Build history of the part. All positions in model axes, mm. Give positions to 0.01 mm unless a question says otherwise; leave off trailing zeros. Order: outer loops, then holes, each group sorted by start corner. A loop starts at its lowest first (then second) coordinate and runs counter-clockwise, first axis right, second up. Notation, with made-up numbers: (73, 11.5) - (132, 11.5) arc R8 ccw to (132, 26.5) - close; hole circle Ø2 at (-36.75, -16.5). An arc over 180 degrees is marked (long way). Answer in a Markdown table with one row per item.
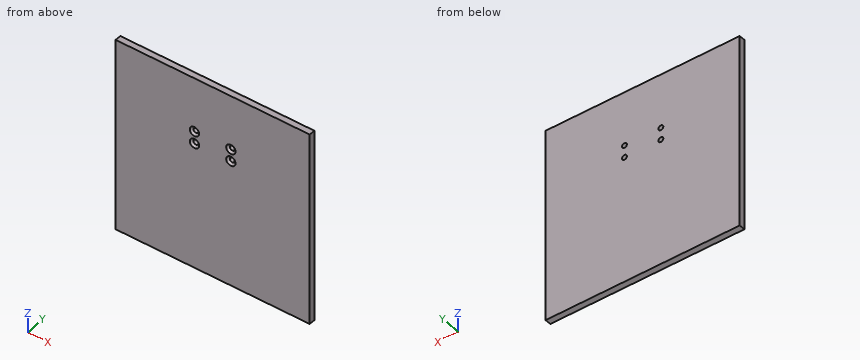
```python
from build123d import *

# Parameters (mm, degrees)
SKETCH2_W                                          = 203.2
SKETCH2_H                                          = 203.2
BOSS_EXTRUDE2_DEPTH                                = 6.35
CSK_FOR_10_FLAT_HEAD_MACHINE_SCREW_100_D           = 5.1054
CSK_FOR_10_FLAT_HEAD_MACHINE_SCREW_100_CSINK_D     = 9.779
CSK_FOR_10_FLAT_HEAD_MACHINE_SCREW_100_CSINK_ANGLE = 100


with BuildPart() as part:
    # Sketch2 → Boss-Extrude2 (new body)
    with BuildSketch(Plane(origin=(0, 0, 0), x_dir=(1, 0, 0), z_dir=(0, 1, 0))):
        with Locations((101.6, 101.6)):
            Rectangle(SKETCH2_W, SKETCH2_H)
    extrude(amount=BOSS_EXTRUDE2_DEPTH)

    # CSK for #10 Flat Head Machine Screw (100)1 (through all)
    with Locations(Plane(origin=(0, 0, 0), x_dir=(-1, 0, 0), z_dir=(0, -1, 0))):
        with Locations((-82.55, 57.15), (-82.55, 69.85), (-120.65, 57.15), (-120.65, 69.85)):
            CounterSinkHole(CSK_FOR_10_FLAT_HEAD_MACHINE_SCREW_100_D / 2, CSK_FOR_10_FLAT_HEAD_MACHINE_SCREW_100_CSINK_D / 2, counter_sink_angle=CSK_FOR_10_FLAT_HEAD_MACHINE_SCREW_100_CSINK_ANGLE)


solid = part.part
```
1. Probe line 1 (Z direction, x = 120.65, y = 4.35); line 2 (X direction, y = 3.4, z = -57.15); line 3 (Z direction, x = 81, y = 3). List the from-to ranges inside material, lowest first.
Check result:
| item | result |
|---|---|
| line 1 | z = -203.2 to -72.4, -67.3 to -59.7, -54.6 to 0 |
| line 2 | x = 0 to 80, 85.1 to 118.1, 123.2 to 203.2 |
| line 3 | z = -203.2 to -71.88, -67.82 to -59.18, -55.12 to 0 |
2. Drop flat-ended pins along their axis: P1, Ø6.5, axis at x = 82.55, z = -69.85, coming from the -Y side; P2, Ø1.5, axis at x = 171, y = 4, coming from the +Z side. Give the stop position or say it passes through.
Check result:
| item | result |
|---|---|
| P1 | stops at y = 1.38 |
| P2 | stops at z = 0 |
3. Cut at A-A on z = -69.85. Write the cut outline in (x, y), and give its area (3 significant figures).
Check result:
| item | result |
|---|---|
| outline | (0, 0) - (77.66, 0) - (80, 1.96) - (80, 6.35) - (0, 6.35) - close; (85.1, 1.96) - (87.44, 0) - (115.76, 0) - (118.1, 1.96) - (118.1, 6.35) - (85.1, 6.35) - close; (123.2, 1.96) - (125.54, 0) - (203.2, 0) - (203.2, 6.35) - (123.2, 6.35) - close |
| area | 1,220 mm² |
4. Cut at B-B on x = 120.65. Write the cut outline in (y, z), and give its area (3 significant figures).
Check result:
| item | result |
|---|---|
| outline | (0, -203.2) - (6.35, -203.2) - (6.35, -72.4) - (1.96, -72.4) - (0, -74.74) - close; (0, -64.96) - (1.96, -67.3) - (6.35, -67.3) - (6.35, -59.7) - (1.96, -59.7) - (0, -62.04) - close; (0, -52.26) - (1.96, -54.6) - (6.35, -54.6) - (6.35, 0) - (0, 0) - close |
| area | 1,220 mm² |
